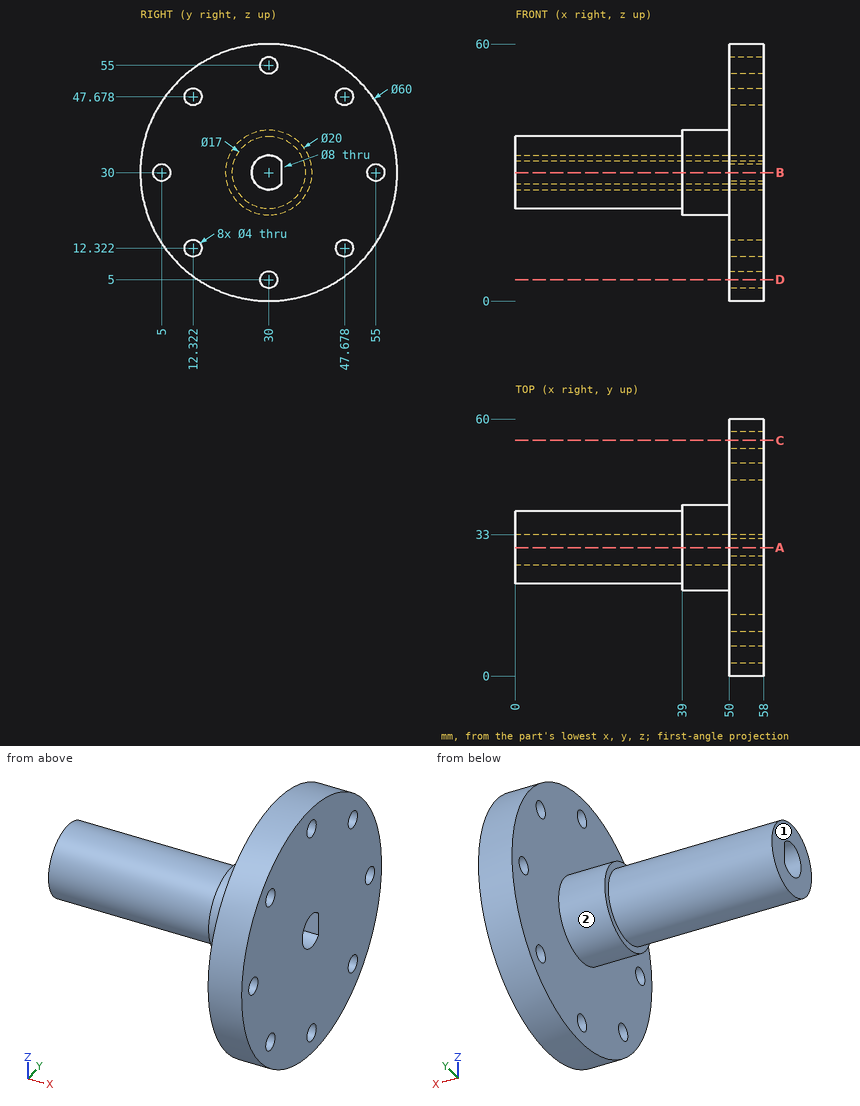
Verification items for this drawing (mm, ordinates from the low corner). A direction names the side the tool comes from. Round coordinates to 2 decimals unless told otherwise and drop trailing zeros. Order: outer loops, then holes, each group sorted by start corner. A loop starts at its lowest first (then second) coordinate and runs counter-clockwise, first axis right, second up. Notation, with made-up numbers: (-38, 51) - (-13, 51) arc R26 cw to (-13, 77) - close; hole circle Ø1 at (-21, -22). An arc over 180 degrees is marked (long way). Answer as CSV lines item,"result". Start each with the question number.
1) Section check C-C (y = 55). Record the cut outline in (x, z).
2) Tool access check on the marked faces 1 and 2. Record the directions out of +Z, -Z, +X, -X, +Y, -Y that give a thin tool (end or side, any length) a straight path to the whole face; none if there is none.
3) Depth check by flat-ended pin: pin 1 (3.5 mm diameter, centred on y = 30, z = 55, fed in from +X); pin 2 (10 mm diameter, centred on x = 35, y = 40, fed in from -Z); pin 3 (1.5 mm diameter, centred on x = 33, y = 30.5, fed in from +Z); pin 4 (4.5 mm diameter, centred on y = 47.68, z = 12.32, fed in from -X). Enter the tip coordinate at first touch or a pass-through.
4) Section check B-B (z = 30). Record the cut outline in (x, y), then the cut area to 3 significant figures.
5) Section check A-A (y = 30). Record the cut outline in (x, z).
6) Scan lines: probe 1 along Y at (x, z) = (54.5, 30); probe 2 along Y at (x, z) = (53.5, 14) (1 decimal); probe 3 along Y at (x, z) = (30, 30). Record each from-to range of solid material in increasing order.
Determined:
1,outline,"(50, 13.42) - (58, 13.42) - (58, 28) - (50, 28) - close; (50, 32) - (58, 32) - (58, 46.58) - (50, 46.58) - close"
2,face 1,"+Z, -Z, -X, +Y, -Y"
2,face 2,"-X"
3,pin 1,"through"
3,pin 2,"z = 22.86"
3,pin 3,"z = 38.5"
3,pin 4,"x = 50"
4,outline,"(0, 21.5) - (39, 21.5) - (39, 20) - (50, 20) - (50, 7) - (58, 7) - (58, 26) - (0, 26) - close; (0, 33) - (58, 33) - (58, 53) - (50, 53) - (50, 40) - (39, 40) - (39, 38.5) - (0, 38.5) - close; (50, 0) - (58, 0) - (58, 3) - (50, 3) - close; (50, 57) - (58, 57) - (58, 60) - (50, 60) - close"
4,area,"893 mm^2"
5,outline,"(0, 21.5) - (39, 21.5) - (39, 20) - (50, 20) - (50, 7) - (58, 7) - (58, 26) - (0, 26) - close; (0, 34) - (58, 34) - (58, 53) - (50, 53) - (50, 40) - (39, 40) - (39, 38.5) - (0, 38.5) - close; (50, 0) - (58, 0) - (58, 3) - (50, 3) - close; (50, 57) - (58, 57) - (58, 60) - (50, 60) - close"
6,probe 1,"0 to 3, 7 to 26, 33 to 53, 57 to 60"
6,probe 2,"4.6 to 11.2, 13.4 to 46.6, 48.8 to 55.4"
6,probe 3,"21.5 to 26, 33 to 38.5"
